Work out the finished part from the listing and answer in its coordinate system (mm). A direction names the side the tool comes from. Round coordinates to 2 decimals unless told otherwise and drop trailing zeros. Order: outer loops, then holes, each group sorted by start corner. A loop starts at its lowest first (then second) coordinate and runs counter-clockwise, first axis right, second up. Notation, with made-up numbers: (76, 1) - (105, 1) arc R12 ccw to (105, 17) - close; hole circle Ø8 at (-15.5, 27). An arc over 180 degrees is marked (long way). Use CSV: the item, a comma, the result in double quotes.
from build123d import *

# Parameters (mm, degrees)
CROQUIS1_W                = 47.2
CROQUIS1_H                = 11.8
CROQUIS1_W_2              = 43.2
CROQUIS1_H_2              = 7.8
SALIENTE_EXTRUIR1_DEPTH   = 20
CROQUIS2_W                = 1.5
CROQUIS2_H                = 1.2
CORTAR_EXTRUIR1_DEPTH     = 20
CROQUIS3_W                = 1
CROQUIS3_H                = 2
SALIENTE_EXTRUIR2_DEPTH   = 20
SALIENTE_EXTRUIR2_2_DEPTH = 20
SALIENTE_EXTRUIR2_3_DEPTH = 20
SALIENTE_EXTRUIR2_4_DEPTH = 20
CROQUIS5_W                = 47.2
CROQUIS5_H                = 11.8
SALIENTE_EXTRUIR3_DEPTH   = 10
CROQUIS6_R                = 0.8
CORTAR_EXTRUIR2_DEPTH     = 10


with BuildPart() as part:
    # Croquis1 → Saliente-Extruir1 (new body)
    with BuildSketch(Plane.XY):
        with Locations((0, -8.96031539)):
            Rectangle(CROQUIS1_W, CROQUIS1_H)
        with Locations((0, -8.96031539)):
            Rectangle(CROQUIS1_W_2, CROQUIS1_H_2, mode=Mode.SUBTRACT)
    extrude(amount=SALIENTE_EXTRUIR1_DEPTH)

    # Croquis2 → Cortar-Extruir1 (cut)
    with BuildSketch(Plane.XY.offset(20)):
        with Locations((-15.35, -4.46031539)):
            Rectangle(CROQUIS2_W, CROQUIS2_H)
        with Locations((15.35, -4.46031539)):
            Rectangle(CROQUIS2_W, CROQUIS2_H)
    extrude(amount=-CORTAR_EXTRUIR1_DEPTH, mode=Mode.SUBTRACT)



with BuildPart() as body_2:
    # Croquis3 → Saliente-Extruir2 (new body)
    with BuildSketch(Plane.XY.offset(20)):
        with Locations((-6.6, -6.06031539)):
            Rectangle(CROQUIS3_W, CROQUIS3_H)
    extrude(amount=-SALIENTE_EXTRUIR2_DEPTH)


with BuildPart() as body_3:
    # Croquis3 → Saliente-Extruir2 2 (new body)
    with BuildSketch(Plane.XY.offset(20)):
        with Locations((6.6, -6.06031539)):
            Rectangle(CROQUIS3_W, CROQUIS3_H)
    extrude(amount=-SALIENTE_EXTRUIR2_2_DEPTH)


with BuildPart() as body_4:
    # Croquis3 → Saliente-Extruir2 3 (new body)
    with BuildSketch(Plane.XY.offset(20)):
        with Locations((-6.6, -11.86031539)):
            Rectangle(CROQUIS3_W, CROQUIS3_H)
    extrude(amount=-SALIENTE_EXTRUIR2_3_DEPTH)


with BuildPart() as body_5:
    # Croquis3 → Saliente-Extruir2 4 (new body)
    with BuildSketch(Plane.XY.offset(20)):
        with Locations((6.6, -11.86031539)):
            Rectangle(CROQUIS3_W, CROQUIS3_H)
    extrude(amount=-SALIENTE_EXTRUIR2_4_DEPTH)


with BuildPart() as part_1:
    add(part.part)

    add(body_2.part)  # Saliente-Extruir3 merges body 2

    add(body_3.part)  # Saliente-Extruir3 merges body 3

    add(body_4.part)  # Saliente-Extruir3 merges body 4

    add(body_5.part)  # Saliente-Extruir3 merges body 5
    # Croquis5 → Saliente-Extruir3 (add)
    with BuildSketch(Plane(origin=(0, 0, 0), x_dir=(-1, 0, 0), z_dir=(0, 0, -1))):
        with Locations((0, -8.96031539)):
            Rectangle(CROQUIS5_W, CROQUIS5_H)
    extrude(amount=SALIENTE_EXTRUIR3_DEPTH)

    # Croquis6 → Cortar-Extruir2 (cut)
    with BuildSketch(Plane.XY):
        with Locations((-4.685466197, -10.055288468)):
            Circle(CROQUIS6_R)
        with Locations((2.49552004, -8.782063958)):
            Circle(CROQUIS6_R)
    extrude(amount=-CORTAR_EXTRUIR2_DEPTH, mode=Mode.SUBTRACT)


solid = part_1.part
(1) Find the intervals of material crossed by L1, parallel to X at y = -5, z = 4.75; L2, parallel to X at y = -7, z = 5.5; L3, parallel to Y at x = -6, z = 15.75, in increasing order. Write a range as from..to.
Findings below:
L1,"x = -23.6..-16.1, -14.6..14.6, 16.1..23.6"
L2,"x = -23.6..-21.6, -7.1..-6.1, 6.1..7.1, 21.6..23.6"
L3,"y = -14.86..-12.86, -5.06..-3.06"
(2) Find section C-C (x = -4.5). Determine the outline of the cut face in (y, z).
Findings below:
outline,"(-14.86, -10) - (-10.83, -10) - (-10.83, 0) - (-12.86, 0) - (-12.86, 20) - (-14.86, 20) - close; (-9.28, -10) - (-3.06, -10) - (-3.06, 20) - (-5.06, 20) - (-5.06, 0) - (-9.28, 0) - close"
(3) Find section B-B (x = 18). Determine the outline of the cut face in (y, z).
Findings below:
outline,"(-14.86, -10) - (-3.06, -10) - (-3.06, 20) - (-5.06, 20) - (-5.06, 0) - (-12.86, 0) - (-12.86, 20) - (-14.86, 20) - close"
(4) For faces 4 (the flat face through (-6.1, -6, 10)), 5 (the cylindrical face through (-3.946, -10.362, -4.93)), determine the directions among +Z, -Z, +X, -X, +Y, -Y from which every point of the face is accessible in a straight line to the end or side of a thin tool.
Findings below:
face 4,"+Z"
face 5,"+Z, -Z"
(5) This flat-tipped pin is pushed along its axis until it touches: pin 1 (7 mm diameter, centred on x = -2, y = -6.5, fed in from +Z). Where does it stop, or does it pass through?
Findings below:
pin 1,"stops at z = 20"
(6) The mould has two halves that part along Y. Classify faces 1 (the flat face through (0, -9, -10)), 2 (the flat face through (-11, -5.06, 10)), 3 (the flat face through (0, -14.86, 5)): released by +Y, released by -Y, zero draft, split by the parting line, or undercut.
Findings below:
face 1,"zero draft"
face 2,"undercut"
face 3,"released by -Y"
